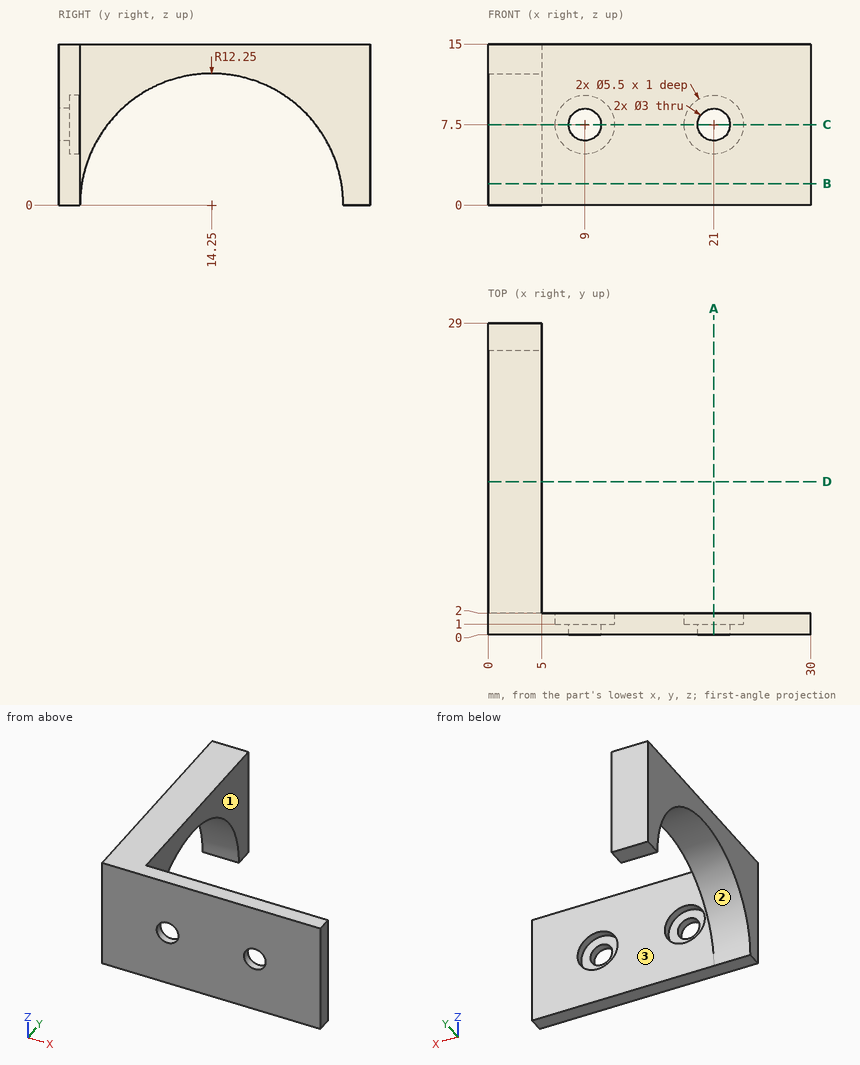
Input: dimensioned drawing with shaded views. Units: mm. Origin: part minimum x, y, z. Coordinates: 2 decimals unless noted, no trailing zeros. Loops run counter-clockwise (first coordinate to the right, second up) from the corner with the lowest first, then second, coordinate; pieces in that order, holes last. Notation, with made-up numbers: M 41.25,-28.5 L 77.25,-28.5 A33 ccw 77.25,-0.5 Z; hole C 47.5,-28 d9. An arc over 180 degrees is marked long. Use a Markdown table: item, result. Add a question column.
Q1. Section query A-A, the plane x = 21. Return loops of the section in (y, z).
Q2. Draft query along Y for the marked faces 1, 2 and 3. Return one class per face: pulls with the +Y half, pulls with the -Y half, needs draft (parallel to the pull), parting line crosses it, or undercut.
Q3. Material intervals for L1, parallel to Z at x = 9, y = 1.3; L2, parallel to Y at x = 13.25, z = 3.75; L3, parallel to X at y = 18.5, z = 13.75, sorted ascending.
Q4. Section query D-D, the plane y = 14.25. Return loops of the section in (x, z).
Q5. Section query B-B, the plane z = 2. Return loops of the section in (x, y).
Q6. Section query C-C, the plane z = 7.5. Return loops of the section in (x, y).
Q7. First-contact query: pin 1 (4.5 mm diameter, centred on x = 21.5, z = 6, fed in from +Y); pin 2 (2.5 mm diameter, centred on x = 8.5, z = 8, fed in from +Y). Flat tips, straight axial feed; report the tip coordinate or a pass-through.
Result:
| question | item | result |
|---|---|---|
| 1 | outline | M 0,0 L 2,0 L 2,4.75 L 1,4.75 L 1,6 L 0,6 Z; M 0,9 L 1,9 L 1,10.25 L 2,10.25 L 2,15 L 0,15 Z |
| 2 | face 1 | needs draft |
| 2 | face 2 | undercut |
| 2 | face 3 | pulls with the +Y half |
| 3 | L1 | z = 0 to 4.75, 10.25 to 15 |
| 3 | L2 | y = 0 to 2 |
| 3 | L3 | x = 0 to 5 |
| 4 | outline | M 0,12.25 L 5,12.25 L 5,15 L 0,15 Z |
| 5 | outline | M 0,0 L 30,0 L 30,2 L 5,2 L 5,2.16 L 0,2.16 Z; M 0,26.34 L 5,26.34 L 5,29 L 0,29 Z |
| 6 | outline | M 0,0 L 7.5,0 L 7.5,1 L 6.25,1 L 6.25,2 L 5,2 L 5,4.56 L 0,4.56 Z; M 0,23.94 L 5,23.94 L 5,29 L 0,29 Z; M 10.5,0 L 19.5,0 L 19.5,1 L 18.25,1 L 18.25,2 L 11.75,2 L 11.75,1 L 10.5,1 Z; M 22.5,0 L 30,0 L 30,2 L 23.75,2 L 23.75,1 L 22.5,1 Z |
| 7 | pin 1 | stops at y = 2 |
| 7 | pin 2 | stops at y = 1 |
